Design review of the part built by this model. Coordinates are the model's own, in mm. Face numbers are marked on the shaded views. Round coordinates to 2 decimals unless told otherwise and drop trailing zeros. Loops run counter-clockwise (first coordinate to the right, second up) from the corner with the lowest first, then second, coordinate; pieces in that order, holes last. Notation, with made-up numbers: M 12.25,-11.5 L 64.25,-11.5 A24 ccw 64.25,15.5 Z; hole C 79.25,-27 d2. An arc over 180 degrees is marked long. Use a Markdown table: item, result.
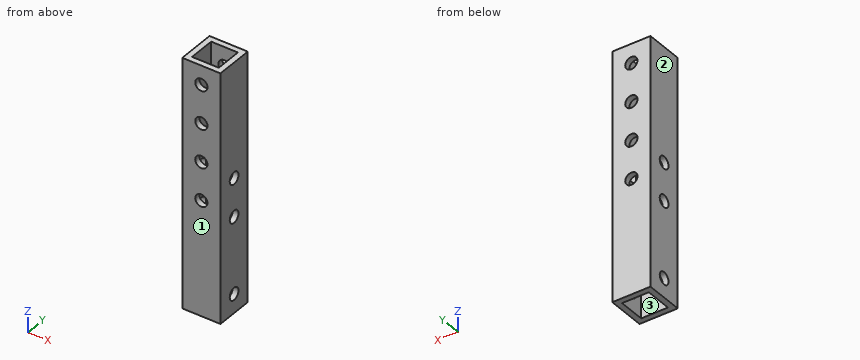
from build123d import *

# Parameters (mm, degrees)
SKETCH_1_W          = 10
SKETCH_1_H          = 10
SKETCH_1_W_2        = 7
SKETCH_1_H_2        = 7
EXTRUDE_1_DEPTH     = 65
SKETCH_3_R          = 1.6
CUT_EXTRUDE_1_DEPTH = 66.954529791
SKETCH_4_R          = 1.6
CUT_EXTRUDE_2_DEPTH = 66.954529791
SKETCH_5_R          = 1.6
CUT_EXTRUDE_3_DEPTH = 66.954529791


with BuildPart() as part:
    # ｽｹｯﾁ1 → 押し出し-薄板1 (new body)
    with BuildSketch(Plane.XY):
        Rectangle(SKETCH_1_W, SKETCH_1_H)
        Rectangle(SKETCH_1_W_2, SKETCH_1_H_2, mode=Mode.SUBTRACT)
    extrude(amount=EXTRUDE_1_DEPTH)

    # ｽｹｯﾁ3 → ｶｯﾄ - 押し出し1 (cut, through all)
    with BuildSketch(Plane.ZY.offset(5)):
        with Locations((5, 0)):
            Circle(SKETCH_3_R)
        with Locations((25, 0)):
            Circle(SKETCH_3_R)
    extrude(amount=-CUT_EXTRUDE_1_DEPTH, mode=Mode.SUBTRACT)

    # ｽｹｯﾁ4 → ｶｯﾄ - 押し出し2 (cut, through all)
    with BuildSketch(Plane.XZ.offset(5)):
        with Locations(Location((0, 30, 0), (0, 0, 270))):
            Circle(SKETCH_4_R)
        with Locations(Location((0, 40, 0), (0, 0, 270))):
            Circle(SKETCH_4_R)
        with Locations(Location((0, 50, 0), (0, 0, 270))):
            Circle(SKETCH_4_R)
        with Locations(Location((0, 60, 0), (0, 0, 270))):
            Circle(SKETCH_4_R)
    extrude(amount=-CUT_EXTRUDE_2_DEPTH, mode=Mode.SUBTRACT)

    # ｽｹｯﾁ5 → ｶｯﾄ - 押し出し3 (cut, through all)
    with BuildSketch(Plane(origin=(5, 0, 0), x_dir=(0, 0, -1), z_dir=(1, 0, 0))):
        with Locations((-35, 0)):
            Circle(SKETCH_5_R)
    extrude(amount=-CUT_EXTRUDE_3_DEPTH, mode=Mode.SUBTRACT)


solid = part.part
1. Take a section at D-D on z = 17. Give the boundary of the cut face in (x, y).
Check values:
| item | result |
|---|---|
| outline | M -5,-5 L 5,-5 L 5,5 L -5,5 Z; hole M -3.5,-3.5 L 3.5,-3.5 L 3.5,3.5 L -3.5,3.5 Z |
2. Take a section at C-C on x = -4.25. Give the boundary of the cut face in (y, z).
Check values:
| item | result |
|---|---|
| outline | M -5,0 L 5,0 L 5,65 L -5,65 Z; hole C 0,5 d3.2; hole C 0,25 d3.2; hole C 0,35 d3.2 |
3. Take a section at B-B on z = 5. Give the boundary of the cut face in (x, y).
Check values:
| item | result |
|---|---|
| outline | M -5,-5 L 5,-5 L 5,-1.6 L 3.5,-1.6 L 3.5,-3.5 L -3.5,-3.5 L -3.5,-1.6 L -5,-1.6 Z; M -5,1.6 L -3.5,1.6 L -3.5,3.5 L 3.5,3.5 L 3.5,1.6 L 5,1.6 L 5,5 L -5,5 Z |
4. The part is to be moulded in two halves that separate along Y. For the marked faces 1, 2 and 3, say which applies: pulls with the +Y half, pulls with the -Y half, needs draft (parallel to the pull), parting line crosses it, or undercut.
Check values:
| item | result |
|---|---|
| face 1 | pulls with the -Y half |
| face 2 | needs draft |
| face 3 | undercut |
5. Take a section at A-A on y = 2.75. Give the boundary of the cut face in (x, z), and give its area (3 significant figures).
Check values:
| item | result |
|---|---|
| outline | M -5,0 L -3.5,0 L -3.5,65 L -5,65 Z; M 3.5,0 L 5,0 L 5,65 L 3.5,65 Z |
| area | 195 mm² |
6. Insertion check: pin 1 (4 mm diameter, centred on y = 0, z = 25, fed in from -X). The pin has a flat end and moves straight along its axis. Give the tip position at first contact, or say it passes through.
Check values:
| item | result |
|---|---|
| pin 1 | stops at x = -5 |
7. Wall thickness on line 1 along Y through (x, z) = (-1.5, 48); line 2 along X through (y, z) = (4.5, 40): over which ranges is each line inside the solid? List them lowest first. Write a range as from..to.
Check values:
| item | result |
|---|---|
| line 1 | y = -5..-3.5, 3.5..5 |
| line 2 | x = -5..-1.6, 1.6..5 |
